Design review of the part built by this model. Coordinates are the model's own, in mm. A direction names the side the tool comes from. Round coordinates to 2 decimals unless told otherwise and drop trailing zeros. Order: outer loops, then holes, each group sorted by start corner. A loop starts at its lowest first (then second) coordinate and runs counter-clockwise, first axis right, second up. Notation, with made-up numbers: (-7, 44.25) - (11, 44.25) arc R19 cw to (11, 58.25) - close; hole circle Ø8 at (-29.5, 17.25). An arc over 180 degrees is marked (long way). Write item = value, one per line.
from build123d import *

# Parameters (mm, degrees)
F0_R     = 3.175
F1_DEPTH = 38.1
F2_R     = 5.08
F3_DEPTH = 38.1


with BuildPart() as f1:
    # F0 (on Front) → F1 (new body)
    with BuildSketch(Plane.XZ):
        with BuildLine():
            ThreePointArc((38.1, 139.7), (0, 177.8), (-38.1, 139.7))
            Line((-38.1, 139.7), (-38.1, -139.7))
            Line((-38.1, -139.7), (38.1, -164.458881))
            Line((38.1, -164.458881), (38.1, -62.858881))
            Line((38.1, -62.858881), (19.05, -62.858881))
            Line((19.05, -62.858881), (19.05, 6.991119))
            Line((19.05, 6.991119), (38.1, 6.991119))
            Line((38.1, 6.991119), (38.1, 139.7))
        make_face()
        with Locations((0, 146.05)):
            Circle(F0_R, mode=Mode.SUBTRACT)
    extrude(amount=F1_DEPTH)

    # F2
    f2_edges = [f1.edges().sort_by_distance(p)[0] for p in [
        (-38.1, 0, 0),
        (38.1, 0, -113.658881),
        (38.1, 0, 73.34556),
        (0, 0, 177.8),
        (-38.1, -38.1, 0),
        (0, -38.1, 177.8),
        (38.1, -38.1, -113.658881),
        (38.1, -38.1, 73.34556),
    ]]
    fillet(f2_edges, radius=F2_R)

    # F0 (on Front) → F3 (cut)
    with BuildSketch(Plane.XZ):
        with Locations((0, 146.05)):
            Circle(F0_R)
    extrude(amount=-F3_DEPTH, mode=Mode.SUBTRACT)


solid = f1.part
1) We need section A-A on y = -17.5. Write out the cut boundary in (x, z) (3 decimals), and give its area (3 significant figures).
Findings:
outline = (-38.1, -139.7) - (38.1, -164.459) - (38.1, -62.859) - (19.05, -62.859) - (19.05, 6.991) - (38.1, 6.991) - (38.1, 139.7) arc R38.1 ccw to (-38.1, 139.7) - close; hole circle Ø6.35 at (0, 146.05)
area = 23,200 mm^2
2) For faces 4 (the flat face through (29, -19, -62.859)), 5 (the flat face through (0, -38.1, 7)), list the 3-axis set-ups (+Z, -Z, +X, -X, +Y, -Y) from which the entire face can be reached by the end or side of a thin tool; tool diameter is ignored.
Findings:
face_4 = +X, +Y, -Y
face_5 = +Z, -Z, +X, -X, -Y
3) We need section B-B on x = 0. Write out the cut boundary in (y, z) (3 decimals).
Findings:
outline = (-38.1, -152.079) - (0, -152.079) - (0, 142.875) - (-38.1, 142.875) - close; (-38.1, 149.225) - (0, 149.225) - (0, 172.72) arc R5.08 ccw to (-5.08, 177.8) - (-33.02, 177.8) arc R5.08 ccw to (-38.1, 172.72) - close
4) The part is to be moulded in two halves that separate along Z. For faces 1 (the flat face through (38.1, -19, 72)), 2 (the cylindrical face through (-0.4, -18.8, 149.2)), 3 (the cylindrical face through (0.84, -18.85, 177.79)), say which applies: released by +Z, released by -Z, zero draft, split by the parting line, or undercut.
Findings:
face_1 = zero draft
face_2 = undercut
face_3 = released by +Z
5) To check wall thickness, follow L1, parallel to X at y = -16, z = 146; L2, parallel to Z at x = 20.5, y = -30; L3, parallel to Z at x = -1, y = -14.5. State the ranges of each line that lie inside material, in increasing order. Write a range as from..to.
Findings:
L1 = -37.58..-3.17, 3.17..37.58
L2 = -158.74..-62.86, 6.99..171.81
L3 = -151.75..143.04, 149.06..177.79
6) Clearance check with flat-ended pins moving along their axes: pin 1 Ø15 at (x, y) = (26, -25) entering from +Z; pin 2 Ø10 at (x, z) = (0, 146.05) entering from -Y; pin 3 Ø12 at (x, y) = (-25.5, -15) entering from +Z; pin 4 Ø1.5 at (x, y) = (-13, -11.5) entering from +Z. State where each tip first meets the part, or that it passes through.
Findings:
pin_1 = 173.01
pin_2 = -38.1
pin_3 = 172.43
pin_4 = 175.78
7) We need section C-C on z = -47. Write out the cut boundary in (x, y), and give its area (3 significant figures).
Findings:
outline = (-38.1, -33.02) arc R5.08 ccw to (-33.02, -38.1) - (19.05, -38.1) - (19.05, 0) - (-33.02, 0) arc R5.08 ccw to (-38.1, -5.08) - close
area = 2,170 mm^2
